from build123d import *

# Parameters (mm, degrees)
SKETCH1_W               = 20
SKETCH1_H               = 20
SKETCH1_W_2             = 18
SKETCH1_H_2             = 18
BOSS_EXTRUDE1_DEPTH     = 10
BOSS_EXTRUDE3_REACH     = 26.495
CUT_EXTRUDE1_DEPTH      = 25.494897428
CUT_EXTRUDE1_DEPTH_BACK = 25.494897428
SKETCH5_R               = 6.1
CUT_EXTRUDE2_DEPTH      = 10


with BuildPart() as part:
    # Sketch1 → Boss-Extrude1 (new body)
    with BuildSketch(Plane.XY):
        Rectangle(SKETCH1_W, SKETCH1_H)
        Rectangle(SKETCH1_W_2, SKETCH1_H_2, mode=Mode.SUBTRACT)
    extrude(amount=BOSS_EXTRUDE1_DEPTH)

    # Sketch3 → Boss-Extrude3 (add, up to next)
    with BuildSketch(Plane(origin=(10, 0, 0), x_dir=(0, 0, -1), z_dir=(1, 0, 0)), mode=Mode.PRIVATE) as boss_extrude3_sk1:
        Polygon((0, 9), (-3.350212633, -10), (-4.365639245, -10), (-1.015426612, 9), align=None)
    boss_extrude3_tool1 = extrude(boss_extrude3_sk1.sketch, amount=-BOSS_EXTRUDE3_REACH, mode=Mode.PRIVATE) - part.part
    add(boss_extrude3_tool1.solids().sort_by_distance((10, -0.5, 2.18282))[0])

    # Sketch4 → Cut-Extrude1 (cut, two sides: drawn at the far end of the back side and taken through both)
    with BuildSketch(Plane.ZY.offset(10).offset(-CUT_EXTRUDE1_DEPTH_BACK)):
        Polygon((-8.537287031, 63.176131209), (0.839099631, 10), (4.365639245, -10), (13.742025907, -63.176131209), (120.094288326, -44.423357885), (97.814975388, 81.928904533), align=None)
    extrude(amount=CUT_EXTRUDE1_DEPTH + CUT_EXTRUDE1_DEPTH_BACK, mode=Mode.SUBTRACT)

    # Sketch5 → Cut-Extrude2 (cut)
    with BuildSketch(Plane(origin=(0, 0.271383206, 1.539090645), x_dir=(-1, 0, 0), z_dir=(0, -0.17364817766692345, -0.9848077530122092))):
        with Locations(Location((0, 0, 0), (0, 0, 90))):
            Circle(SKETCH5_R)
    extrude(amount=-CUT_EXTRUDE2_DEPTH, mode=Mode.SUBTRACT)


solid = part.part
CAD build for the part. Positions are in the model's coordinates, mm. A direction names the side the tool comes from. Coordinates: 2 decimals unless noted, no trailing zeros. Loops run counter-clockwise (first coordinate to the right, second up) from the corner with the lowest first, then second, coordinate; pieces in that order, holes last. Notation, with made-up numbers: (-38, 53.5) - (-13, 53.5) arc R18 cw to (-13, 67.5) - close; hole circle Ø4 at (67.25, -3.75). An arc over 180 degrees is marked (long way). Write item = value, one per line. Start each with the question number.
Q1. Drill centre lines: L1, parallel to X at y = -4, z = 1; L2, parallel to Y at x = -0.5, z = 2.5; L3, parallel to X at y = -5, z = 2.55. Where is each one in solid material? Low to high.
Q2. Cut at C-C, the plane y = 8. List the corners of the cut face in (x, z), then the cut area to 3 significant figures.
Q3. Pull direction Y, two halves, no side cores. Call faces 3 (the flat face through (-0.8, -9.6, 0)), 4 (the flat face through (-0.1, 10, 0.4)), 5 (the flat face through (0, -9, 2)): pulls with the +Y half, pulls with the -Y half, needs draft (parallel to the pull), parting line crosses it, or undercut.
Q4. Cut at B-B, the plane x = 6.5. List the corners of the cut face in (y, z).
Q5. Flat gauge pins, fed straight in: pin 1 Ø12 at (x, y) = (-6.5, 6) entering from -Z; pin 2 Ø1.5 at (x, y) = (2.5, 5.5) entering from -Z; pin 3 Ø4 at (x, y) = (3, -7.5) entering from +Z; pin 4 Ø8 at (x, y) = (7, 2) entering from +Z (3 decimals). Where does each tip first touch, or does it go through?
Q6. Cut at D-D, the plane x = -1.5. List the corners of the cut face in (y, z), then the cut area to 3 significant figures.
Q7. Which spindle directions (+Z, -Z, +X, -X, +Y, -Y) get a long thin tool onto all of the face, cutting with end or side? Do faces 1 (the flat face through (6.126, -1.874, 1.917)), 2 (the flat face through (10, -2, 2)). Say none if no direction does.
Q8. Cut at A-A, the plane x = -3.75. List the corners of the cut face in (y, z).
Computed:
q1.L1 = -10 to -9, 9 to 10
q1.L2 = -10 to -9
q1.L3 = -10 to -2.9, 2.9 to 10
q2.outline = (-10, 0) - (-9, 0) - (-9, 0.18) - (9, 0.18) - (9, 0) - (10, 0) - (10, 1.19) - (-10, 1.19) - close
q2.area = 20.7 mm²
q3.face_3 = needs draft
q3.face_4 = pulls with the +Y half
q3.face_5 = undercut
q4.outline = (-10, 0) - (-9, 0) - (-9, 3.17) - (9, 0) - (10, 0) - (10, 0.84) - (-10, 4.37) - close
q5.pin_1 = 0
q5.pin_2 = 0.48
q5.pin_3 = 4.28
q5.pin_4 = 2.955
q6.outline = (-10, 0) - (-9, 0) - (-9, 3.17) - (-5.55, 2.57) - (-5.38, 3.55) - (-10, 4.37) - close; (6.09, 0.51) - (9, 0) - (10, 0) - (10, 0.84) - (6.27, 1.5) - close
q6.area = 11.7 mm²
q7.face_1 = -Z
q7.face_2 = +Z, -Z, +X, +Y, -Y
q8.outline = (-10, 0) - (-9, 0) - (-9, 3.17) - (-4.47, 2.37) - (-4.29, 3.36) - (-10, 4.37) - close; (5.01, 0.7) - (9, 0) - (10, 0) - (10, 0.84) - (5.18, 1.69) - close
